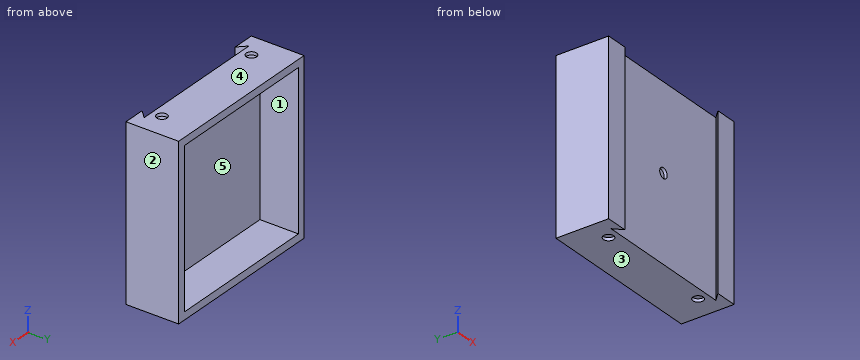
```python
from build123d import *

# Parameters (mm, degrees)
PAD_DEPTH       = 42
SKETCH001_R     = 2.5
POCKET_DEPTH    = 1.5
SKETCH002_W     = 76.5
SKETCH002_H     = 76.5
POCKET001_DEPTH = 19
SKETCH003_R     = 2.55
POCKET002_DEPTH = 1.5


with BuildPart() as part:
    # Sketch (on XY_Plane of Origin) → Pad (new body, symmetric)
    with BuildSketch(Plane.XY):
        Polygon((-42, 22.1), (-42, -3.9), (-31.199999, -3.9), (-35.1, 0), (0, 0), (0, 22.1), align=None)
    extrude(amount=PAD_DEPTH, both=True)

    # Mirrored: part across YZ


with BuildPart() as part_1:
    add(part.part)
    add(part.part.mirror(Plane.YZ))

    # Sketch001 (on Face10 of Mirrored) → Pocket (cut)
    with BuildSketch(Plane.XZ):
        Circle(SKETCH001_R)
    extrude(amount=-POCKET_DEPTH, mode=Mode.SUBTRACT)

    # Sketch002 (on Face2 of Pocket) → Pocket001 (cut)
    with BuildSketch(Plane(origin=(0, 22.1, 0), x_dir=(-1, 0, 0), z_dir=(0, 1, 0))):
        Rectangle(SKETCH002_W, SKETCH002_H)
    extrude(amount=-POCKET001_DEPTH, mode=Mode.SUBTRACT)

    # Sketch003 (on Face5 of Pocket001) → Pocket002 (cut)
    with BuildSketch(Plane.XY.offset(42)):
        with Locations((-30, 5)):
            Circle(SKETCH003_R)
        with Locations((30, 5)):
            Circle(SKETCH003_R)
    pocket002 = extrude(amount=-POCKET002_DEPTH, mode=Mode.SUBTRACT)

    # Mirrored001: Pocket002 across XY
    add(pocket002.mirror(Plane.XY), mode=Mode.SUBTRACT)


solid = part_1.part
```
Can you work these out from the model? Positions are in its coordinate system, mm. Face numbers are marked on the shaded views. A direction names the side the tool comes from. Round coordinates to 2 decimals unless told otherwise and drop trailing zeros. Order: outer loops, then holes, each group sorted by start corner. A loop starts at its lowest first (then second) coordinate and runs counter-clockwise, first axis right, second up.
(1) If I drill on L1, parallel to X at y = 16.5, z = -10.5; L2, parallel to Z at x = 0, y = 0.4, over which ranges is the centre line in solid material (lowest first)?
Results are:
L1: x = -42 to -38.25, 38.25 to 42
L2: z = -42 to -2.5, 2.5 to 42
(2) I'm going to push flat-ended pins straight in: pin 1 (2 mm diameter, centred on x = -5.5, z = 25.5, fed in from +Y); pin 2 (4.5 mm diameter, centred on x = -30, y = 5, fed in from +Z); pin 3 (1.5 mm diameter, centred on x = -30, y = 4.5, fed in from -Z). Where does each tip first touch, or does it pass through?
Results are:
pin 1: stops at y = 3.1
pin 2: stops at z = 40.5
pin 3: stops at z = -40.5
(3) If we section it at C-C (x = 22): Please give me the cut outline in (y, z), plus the area to 3 significant figures.
Results are:
outline: (0, -42) - (22.1, -42) - (22.1, -38.25) - (3.1, -38.25) - (3.1, 38.25) - (22.1, 38.25) - (22.1, 42) - (0, 42) - close
area: 403 mm2
(4) If we section it at B-B (z = 0): Please give me the cut outline in (x, y), plus the area to 3 significant figures.
Results are:
outline: (-42, -3.9) - (-31.2, -3.9) - (-35.1, 0) - (-2.5, 0) - (-2.5, 1.5) - (2.5, 1.5) - (2.5, 0) - (35.1, 0) - (31.2, -3.9) - (42, -3.9) - (42, 22.1) - (38.25, 22.1) - (38.25, 3.1) - (-38.25, 3.1) - (-38.25, 22.1) - (-42, 22.1) - close
area: 464 mm2
(5) On a 3-axis mill with a long thin cutter (end or side, diameter ignored), from which of +Z, -Z, +X, -X, +Y, -Y can I reach the whole of each face in a straight line? I mean the marked faces 4 and 5. Say none if no direction works.
Results are:
face 4: +Z, +X, -X, +Y, -Y
face 5: +Y
(6) If we section it at A-A (y = 10.5): Please give me the cut outline in (x, z), plus the area to 3 significant figures.
Results are:
outline: (-42, -42) - (42, -42) - (42, 42) - (-42, 42) - close; hole (-38.25, -38.25) - (38.25, -38.25) - (38.25, 38.25) - (-38.25, 38.25) - close
area: 1,200 mm2
(7) We'd pull the mould along X, two halves only. Please class the marked faces 1, 2 and 3: +X half, -X half, draft (parallel to the pull), parting line (faces both ways), or undercut.
Results are:
face 1: undercut
face 2: +X half
face 3: draft
(8) If we section it at D-D (y = 5): Please give me the cut outline in (x, z).
Results are:
outline: (-42, -42) - (-32.55, -42) - (-32.55, -40.5) - (-27.45, -40.5) - (-27.45, -42) - (27.45, -42) - (27.45, -40.5) - (32.55, -40.5) - (32.55, -42) - (42, -42) - (42, 42) - (32.55, 42) - (32.55, 40.5) - (27.45, 40.5) - (27.45, 42) - (-27.45, 42) - (-27.45, 40.5) - (-32.55, 40.5) - (-32.55, 42) - (-42, 42) - close; hole (-38.25, -38.25) - (38.25, -38.25) - (38.25, 38.25) - (-38.25, 38.25) - close
